from build123d import *
from OCP.BRepAlgoAPI import BRepAlgoAPI_Cut
from OCP.TopTools import TopTools_ListOfShape

# Parameters (mm, degrees)
SKETCH1_W              = 66
SKETCH1_H              = 28.2
BOSS_EXTRUDE1_DEPTH    = 2
SKETCH5_R              = 1.0500000000000005
BOSS_EXTRUDE2_DEPTH    = 5
SKETCH8_W              = 1.7595642605370743
SKETCH8_H              = 1.7595642605370756
CUT_EXTRUDE3_DEPTH     = 5
FILLET4_R              = 0.2
LPATTERN1_COUNT        = 8
LPATTERN1_PITCH        = 5
LPATTERN1_2_COUNT      = 8
LPATTERN1_2_PITCH      = 5
FILLET4_OF_LPATTERN1_R = 0.2
CUT_EXTRUDE1_DEPTH     = 44.54870836201689
FILLET5_R              = 1.5
BOSS_EXTRUDE3_DEPTH    = 1


with BuildPart() as part:
    # Sketch1 → Boss-Extrude1 (new body)
    with BuildSketch(Plane.XY):
        Rectangle(SKETCH1_W, SKETCH1_H)
    extrude(amount=BOSS_EXTRUDE1_DEPTH)


with BuildPart() as body_2:
    # Sketch5 → Boss-Extrude2 (new body)
    with BuildSketch(Plane.ZY.offset(33)):
        with BuildLine():
            Line((0.5, 15.599999999999998), (0, 14.099999999999998))
            Line((0, 14.099999999999998), (2, 14.099999999999998))
            ThreePointArc((2, 14.099999999999998), (3.0606601717798214, 16.66066017177982), (0.5, 15.599999999999998))
        make_face()
        with Locations((2, 15.599999999999998)):
            Circle(SKETCH5_R, mode=Mode.SUBTRACT)
    boss_extrude2 = extrude(amount=-BOSS_EXTRUDE2_DEPTH)

    # Sketch8 → Cut-Extrude3 (cut)
    with BuildSketch(Plane.ZY.offset(33)):
        with Locations((3.068777942853419, 16.780207609912114)):
            Rectangle(SKETCH8_W, SKETCH8_H)
    cut_extrude3 = extrude(amount=-CUT_EXTRUDE3_DEPTH, mode=Mode.SUBTRACT)

    # Fillet4
    fillet4_edges = [body_2.edges().sort_by_distance(p)[0] for p in [
        (-30.5, 16.632850706939475, 2.1889958125848823),
        (-30.5, 15.900425479643578, 3.006103638389667),
        (-30.5, 17.08804589405884, 2.1889958125848823),
        (-30.5, 15.900425479643578, 3.4696069308427098),
    ]]
    fillet(fillet4_edges, radius=FILLET4_R)


with BuildPart() as part_1:
    add(part.part)

    add(body_2.part)  # LPattern1 merges body 2
    # LPattern1: Boss-Extrude2 ×8, 3 skipped
    with Locations(*[(i * LPATTERN1_PITCH, 0, 0) for i in range(1, LPATTERN1_COUNT) if i not in (2, 4, 6)]):
        add(boss_extrude2)

    # LPattern1 2: Cut-Extrude3 ×8, 3 skipped
    with Locations(*[(i * LPATTERN1_2_PITCH, 0, 0) for i in range(1, LPATTERN1_2_COUNT) if i not in (2, 4, 6)]):
        add(cut_extrude3, mode=Mode.SUBTRACT)

    # Fillet4 of LPattern1
    fillet4_of_lpattern1_edges = [part_1.edges().sort_by_distance(p)[0] for p in [
        (-25.5, 16.632850706939475, 2.1889958125848823),
        (-25.5, 15.900425479643578, 3.006103638389667),
        (-25.5, 17.08804589405884, 2.1889958125848823),
        (-25.5, 15.900425479643578, 3.4696069308427098),
        (-15.5, 16.632850706939475, 2.1889958125848823),
        (-15.5, 15.900425479643578, 3.006103638389667),
        (-15.5, 17.08804589405884, 2.1889958125848823),
        (-15.5, 15.900425479643578, 3.4696069308427098),
        (-5.5, 16.632850706939475, 2.1889958125848823),
        (-5.5, 15.900425479643578, 3.006103638389667),
        (-5.5, 17.08804589405884, 2.1889958125848823),
        (-5.5, 15.900425479643578, 3.4696069308427098),
        (4.5, 16.632850706939475, 2.1889958125848823),
        (4.5, 15.900425479643578, 3.006103638389667),
        (4.5, 17.08804589405884, 2.1889958125848823),
        (4.5, 15.900425479643578, 3.4696069308427098),
    ]]
    fillet(fillet4_of_lpattern1_edges, radius=FILLET4_OF_LPATTERN1_R)


with BuildPart() as cut_extrude1_tool:
    # Sketch6 → Cut-Extrude1 (new, through all)
    with BuildSketch(Plane(origin=(0, 14.099999999999998, 0), x_dir=(1, 0, 0), z_dir=(0, 1, 0))):
        Polygon((-33, 0), (-28, 0), (-28, -7.434056861178039), (-33, -7.434056861178038), align=None)
    extrude(amount=CUT_EXTRUDE1_DEPTH)


with BuildPart() as part_2:
    add(part_1.part)

    # Cut-Extrude1: cut by cut_extrude1_tool, with a tolerance
    cut_extrude1_stock = TopTools_ListOfShape()
    cut_extrude1_stock.Append(part_2.part.wrapped)
    cut_extrude1_tools = TopTools_ListOfShape()
    cut_extrude1_tools.Append(cut_extrude1_tool.part.wrapped)
    cut_extrude1_cut = BRepAlgoAPI_Cut()
    cut_extrude1_cut.SetArguments(cut_extrude1_stock)
    cut_extrude1_cut.SetTools(cut_extrude1_tools)
    cut_extrude1_cut.SetFuzzyValue(0.00001)
    cut_extrude1_cut.Build()
    add(Compound.cast(cut_extrude1_cut.Shape()).solids(), mode=Mode.REPLACE)

    # Fillet5
    fillet5_edges = [part_2.edges().sort_by_distance(p)[0] for p in [
        (0, -14.100000000000001, 0),
        (-33, -1.78e-15, 0),
        (33, -1.78e-15, 0),
    ]]
    fillet(fillet5_edges, radius=FILLET5_R)

    # Sketch9 → Boss-Extrude3 (add)
    with BuildSketch(Plane.XY.offset(2)):
        Polygon((-31.7, 11.599999999999998), (-30.7, 11.599999999999998), (-30.699999999999996, -11.85000000000001), (30.7, -11.85000000000001), (30.7, 11.599999999999994), (31.7, 11.599999999999996), (31.7, -11.850000000000012), (31.700000000000006, -12.850000000000001), (-30.7, -12.85000000000001), (-31.7, -12.850000000000009), align=None)
    extrude(amount=BOSS_EXTRUDE3_DEPTH)


solid = part_2.part
Check sheet for the modelled part. Datum: model origin and axes. Units: mm. A direction names the side the tool comes from. Give positions to 0.01 mm unless a question says otherwise; leave off trailing zeros. Write each loop counter-clockwise with the first axis right and the second up, starting at its lowest first coordinate (ties: lowest second). Pieces come first, ordered by that corner, then holes. Notation, with made-up numbers: (-8.5, 18.25) -> (44.5, 18.25) arc R7 cw to (44.5, 27.25) -> close; hole circle Ø11 at (-30, 25). An arc over 180 degrees is marked (long way). Use one line per item in the form item = value. Start each with the question number.
1. Section check A-A (y = -2.5). Record the cut outline in (x, z).
2. Section check B-B (x = -2). Record the cut outline in (y, z), and give its area (3 significant figures).
3. Section check C-C (x = -15). Record the cut outline in (y, z).
4. Thickness scan on line 1 along Z through (x, y) = (5.75, 15.6); line 2 along X through (y, z) = (-11.5, 2.2); line 3 along X through (y, z) = (-11, 1.3). Record the ranges inside material, lowest first. Write a range as from..to.
5. Mould release check, pull along Y, two halves, no side actions. Record for faces 1 (the cylindrical face through (-25.54, 14.57, 3.09)), 2 (the flat face through (7, 15, 0.9)), 3 (the cylindrical face through (-15.54, 16.67, 0.95)): pulls with the +Y half, pulls with the -Y half, needs draft (parallel to the pull), parting line crosses it, or undercut.
6. Access from +Z, -Z, +X, -X, +Y, -Y to the whole of each face (thin tool, end or side, straight path). Record for faces 4 (the cylindrical face through (-25.54, 16.67, 0.95)), 5 (the cylindrical face through (-5.54, 14.57, 3.09)), 6 (the flat face through (0.1, -12.3, 3)), 7 (the cylindrical face through (0.46, -13.65, 0.43)), 8 (the flat face through (-23, 15, 0.9)).
7. Go/stop test with flat-tipped pins: P1, Ø8, axis at x = 22.5, y = 6.5, coming from the +Z side; P2, Ø0.6, axis at x = -19.5, z = 1, coming from the +Y side; P3, Ø2, axis at y = 4, z = 1, coming from the +X side; P4, Ø0.5, axis at y = 0, z = 2.5, coming from the +X side. Record where each tip stops, or that it passes through.
Conclusion:
q1.outline = (-33, 1.5) arc R1.5 ccw to (-31.5, 0) -> (31.5, 0) arc R1.5 ccw to (33, 1.5) -> (33, 2) -> (31.7, 2) -> (31.7, 3) -> (30.7, 3) -> (30.7, 2) -> (-30.7, 2) -> (-30.7, 3) -> (-31.7, 3) -> (-31.7, 2) -> (-33, 2) -> close
q2.outline = (-14.1, 1.5) arc R1.5 ccw to (-12.6, 0) -> (14.1, 0) -> (14.1, 2) -> (-11.85, 2) -> (-11.85, 3) -> (-12.85, 3) -> (-12.85, 2) -> (-14.1, 2) -> close
q2.area = 56.9 mm²
q3.outline = (-14.1, 1.5) arc R1.5 ccw to (-12.6, 0) -> (14.1, 0) -> (15.6, 0.5) arc R1.5 ccw to (17.1, 1.99) arc R0.2 ccw to (16.9, 2.19) -> (16.85, 2.19) arc R0.2 ccw to (16.65, 1.99) arc R1.05 cw (long way) to (15.68, 3.05) arc R0.2 ccw to (15.9, 3.25) -> (15.9, 3.3) arc R0.2 ccw to (15.72, 3.5) arc R1.5 ccw to (14.1, 2) -> (-11.85, 2) -> (-11.85, 3) -> (-12.85, 3) -> (-12.85, 2) -> (-14.1, 2) -> close
q4.line_1 = 0.5..0.95, 3.05..3.5
q4.line_2 = -31.7..-30.7, 30.7..31.7
q4.line_3 = -32.99..32.99
q5.face_1 = undercut
q5.face_2 = needs draft
q5.face_3 = pulls with the +Y half
q6.face_4 = -Z, +X, -X, +Y
q6.face_5 = +Z, +X, -X
q6.face_6 = +Z, +X, -X, -Y
q6.face_7 = -Z, +X, -X, -Y
q6.face_8 = +Z, -Z, +Y
q7.P1 = 2
q7.P2 = 14.1
q7.P3 = 33
q7.P4 = 31.7
